Design review of the part built by this model. Coordinates are the model's own, in mm. A direction names the side the tool comes from. Coordinates: 2 decimals unless noted, no trailing zeros. Loops run counter-clockwise (first coordinate to the right, second up) from the corner with the lowest first, then second, coordinate; pieces in that order, holes last. Notation, with made-up numbers: (22, 2) - (47, 2) arc R37 ccw to (47, 41) - close; hole circle Ø4 at (3.5, 11.25). An arc over 180 degrees is marked (long way). Answer in a Markdown table with one row per item. Add a question column.
(1) We need section A-A, the plane x = 3.75. Write out the cut boundary in (y, z).
(2) We need section C-C, the plane z = -9.5. Write out the cut boundary in (x, y).
(3) To check wall thickness, follow L1, parallel to Z at x = -1.25, y = 2; L2, parallel to Z at x = 3.25, y = 181. State the ranges of each line that lie inside material, in increasing order. Write a range as [from, to].
(4) The part is to be moulded in two halves that separate along Y. For faces 3 (the face through (0, -1.5, 4)), 4 (the face through (5.5, 110, -13)), 5 (the face through (0, 1.5, 4)), 6 (the face through (-0.08, -9.12, 3.51)), say which applies: released by +Y, released by -Y, zero draft, split by the parting line, or undercut.
(5) We need section B-B, the plane y = 116.5. Write out the cut boundary in (x, z).
(6) For faces 1 (the face through (0, 2, 0)), 2 (the face through (-0.077, 121.542, -10.464)), list the 3-axis set-ups (+Z, -Z, +X, -X, +Y, -Y) from which the entire face can be reached by the end or side of a thin tool; tool diameter is ignored.
(7) Clearance check with flat-ended pins moving along their axes: pin 1 (2.5 mm diameter, centred on x = 1, y = 0.5, fed in from -Z); pin 2 (1 mm diameter, centred on x = -0.5, y = 167, fed in from +Z); pin 3 (3 mm diameter, centred on x = -0.5, z = 2.5, fed in from -Y); pin 4 (1.5 mm diameter, centred on x = -2, y = 176.5, fed in from -Z). State where each tip first meets the part, or that it passes through.
from build123d import *

# Parameters (mm, degrees)
SKETCH3_W                = 11
SKETCH3_H                = 21
BOSS_EXTRUDE1_DEPTH      = 10
CUT_EXTRUDE1_DEPTH       = 8
CUT_EXTRUDE5_DEPTH       = 8
CUT_EXTRUDE5_DEPTH_BACK  = 8
BOSS_EXTRUDE2_DEPTH      = 5.5
BOSS_EXTRUDE2_DEPTH_BACK = 5.5


with BuildPart() as part:
    # Sketch3 → Boss-Extrude1 (new body)
    with BuildSketch(Plane.XY):
        Rectangle(SKETCH3_W, SKETCH3_H)
    extrude(amount=BOSS_EXTRUDE1_DEPTH)

    # Sketch5 → Cut-Extrude1 (cut)
    with BuildSketch(Plane.XY):
        Polygon((0, 1.5), (-2, 1.5), (-2, -1.5), (2, -1.5), (2, 1.5), align=None)
    extrude(amount=CUT_EXTRUDE1_DEPTH, mode=Mode.SUBTRACT)

    # Sketch6 → Cut-Extrude5 (cut, two sides: drawn at the far end of the back side and taken through both)
    with BuildSketch(Plane(origin=(0, 0, 0), x_dir=(0, 0, -1), z_dir=(1, 0, 0)).offset(-CUT_EXTRUDE5_DEPTH_BACK)):
        Polygon((-1.0867085, -10.5), (-6.011599163, -7.693477847), (-8.753565317, 0), (-10, 10.5), (-10, -10.5), (-10, -11.324459918), (-1.0867085, -10.760658811), align=None)
    extrude(amount=CUT_EXTRUDE5_DEPTH + CUT_EXTRUDE5_DEPTH_BACK, mode=Mode.SUBTRACT)

    # Sketch18 → Boss-Extrude2 (add, two sides: drawn at the far end of the back side and taken through both)
    with BuildSketch(Plane(origin=(0, 0, 0), x_dir=(0, 0, -1), z_dir=(1, 0, 0)).offset(-BOSS_EXTRUDE2_DEPTH_BACK)):
        Polygon((0, 10.5), (40.195441972, 227.697760834), (30.362408276, 229.51749937), (-10, 10.5), align=None)
    extrude(amount=BOSS_EXTRUDE2_DEPTH + BOSS_EXTRUDE2_DEPTH_BACK)


solid = part.part
Responses:
| question | item | result |
|---|---|---|
| 1 | outline | (-10.5, 0) - (10.5, 0) - (227.7, -40.2) - (229.52, -30.36) - (10.5, 10) - (0, 8.75) - (-7.69, 6.01) - (-10.5, 1.09) - close |
| 2 | outline | (-5.5, 61.83) - (5.5, 61.83) - (5.5, 116.31) - (-5.5, 116.31) - close |
| 3 | L1 | z = [0, 8.99] |
| 3 | L2 | z = [-31.55, -21.42] |
| 4 | face 3 | undercut |
| 4 | face 4 | zero draft |
| 4 | face 5 | undercut |
| 4 | face 6 | released by -Y |
| 5 | outline | (-5.5, -19.62) - (5.5, -19.62) - (5.5, -9.53) - (-5.5, -9.53) - close |
| 6 | face 1 | -Z, +X, -X, -Y |
| 6 | face 2 | +Z, +X, -X, +Y |
| 7 | pin 1 | stops at z = 0 |
| 7 | pin 2 | stops at z = -18.75 |
| 7 | pin 3 | stops at y = -10.5 |
| 7 | pin 4 | stops at z = -30.86 |
